Can you work these out from the model? Positions are in its coordinate system, mm. Face numbers are marked on the shaded views. A direction names the side the tool comes from. Round coordinates to 2 decimals unless told otherwise and drop trailing zeros. Write each loop counter-clockwise with the first axis right and the second up, starting at its lowest first coordinate (ties: lowest second). Pieces come first, ordered by that corner, then holes. Notation, with made-up numbers: M -38.75,-4.5 L -12.75,-4.5 A33 cw -12.75,31.5 Z; hole C -30.75,52 d6. An arc over 180 degrees is marked long. Answer in a Markdown table with one row per item. Add a question column.
(1) Suppose I cut it at C-C, the plane y = -15.25. Write out the boundary of the cut face in (x, z).
(2) For the marked faces 1, 2 and 3, which set-ups out of +Z, -Z, +X, -X, +Y, -Y let a thin tool reach every point of the face, with its end or its side?
(3) I'm going to push flat-ended pins straight in: pin 1 (8 mm diameter, centred on x = 5.5, z = -26.5, fed in from +Y); pin 2 (7 mm diameter, centred on x = -28, z = 20, fed in from +Y); pin 3 (11.5 mm diameter, centred on x = -29.5, z = -23.5, fed in from +Y); pin 4 (3 mm diameter, centred on y = -10, z = 0, fed in from +X). Where does each tip first touch, or does it pass through?
(4) Suppose I cut it at B-B, the plane x = -32. Write out the boundary of the cut face in (y, z), then the cut area to 3 significant figures.
(5) Suppose I cut it at D-D, the plane z = -13.5. Write out the boundary of the cut face in (x, y), then the cut area to 3 significant figures.
(6) Suppose I cut it at A-A, the plane x = -20. Write out the boundary of the cut face in (y, z), then the cut area to 3 significant figures.
(7) If I drill on probe 1 along Z at (x, y) = (25, -1.3); probe 2 along X at (y, z) = (-8, 1); probe 3 along X at (y, z) = (-12.75, -7), over which ranges is the centre line in solid material (lowest first)?
(8) If we mould it in two halves opening along X, with no side actions, what happens to the marked faces 4, 5 and 6? For each: released by +X, released by -X, zero draft, split by the parting line, or undercut.
from build123d import *

# Parameters (mm, degrees)
SKETCH1_W                        = 70
SKETCH1_H                        = 40
BOSS_EXTRUDE1_DEPTH              = 6.5
SKETCH2_W                        = 100
SKETCH2_H                        = 60
BOSS_EXTRUDE2_DEPTH              = 10
M3_CLEARANCE_HOLE1_D             = 3.2
SKETCH40_R                       = 3
CUT_EXTRUDE10_DEPTH              = 13.5
SKETCH7_W                        = 106.84
SKETCH7_H                        = 66.84
SKETCH7_W_2                      = 100
SKETCH7_H_2                      = 60
BOSS_EXTRUDE3_DEPTH              = 3
CUT_EXTRUDE2_DEPTH               = 1.25
M3_CLEARANCE_HOLE3_D             = 3.2
M3_CLEARANCE_HOLE3_DEPTH         = 12
M3_CLEARANCE_HOLE3_TIP           = 0.96137699
SKETCH23_W                       = 6.48
SKETCH23_H                       = 3
BOSS_EXTRUDE5_DEPTH              = 10
SKETCH26_W                       = 3.2639
SKETCH26_H                       = 13
F_1_4_CLEARANCE_HOLE2_AT_2_COUNT = 2
F_1_4_CLEARANCE_HOLE2_AT_2_PITCH = 45
SKETCH41_W                       = 35
SKETCH41_H                       = 40
SKETCH41_W_2                     = 10
SKETCH41_W_3                     = 5
CUT_EXTRUDE11_DEPTH              = 6.5
SKETCH42_W                       = 15
SKETCH42_H                       = 35
SKETCH42_W_2                     = 10
SKETCH42_H_2                     = 40
CUT_EXTRUDE12_DEPTH              = 7
CUT_EXTRUDE13_DEPTH              = 1.25
M3_CLEARANCE_HOLE5_D             = 3.2
M3_CLEARANCE_HOLE5_DEPTH         = 10
M3_CLEARANCE_HOLE5_TIP           = 0.96137699
FILLET1_R                        = 2
FILLET2_R                        = 1


with BuildPart() as part:
    # Sketch1 → Boss-Extrude1 (new body)
    with BuildSketch(Plane(origin=(0, 0, 0), x_dir=(1, 0, 0), z_dir=(0, 1, 0))):
        Rectangle(SKETCH1_W, SKETCH1_H)
    extrude(amount=-BOSS_EXTRUDE1_DEPTH)

    # Sketch2 → Boss-Extrude2 (add)
    with BuildSketch(Plane.XZ.offset(6.5)):
        with Locations((10, 0)):
            Rectangle(SKETCH2_W, SKETCH2_H)
    extrude(amount=BOSS_EXTRUDE2_DEPTH)

    # M3 Clearance Hole1 (through all)
    with Locations(Plane(origin=(0, 0, 0), x_dir=(1, 0, 0), z_dir=(0, 1, 0))):
        with Locations((-20, 7), (25, 7), (-20, -7), (25, -7)):
            Hole(M3_CLEARANCE_HOLE1_D / 2)

    # Sketch40 → Cut-Extrude10 (cut)
    with BuildSketch(Plane.XZ.offset(16.5)):
        with Locations(Location((-20, 7, 0), (0, 0, 270))):
            Circle(SKETCH40_R)
        with Locations(Location((-20, -7, 0), (0, 0, 270))):
            Circle(SKETCH40_R)
        with Locations(Location((25, 7, 0), (0, 0, 270))):
            Circle(SKETCH40_R)
        with Locations(Location((25, -7, 0), (0, 0, 270))):
            Circle(SKETCH40_R)
    extrude(amount=-CUT_EXTRUDE10_DEPTH, mode=Mode.SUBTRACT)

    # Sketch7 → Boss-Extrude3 (add)
    with BuildSketch(Plane.XZ.offset(16.5)):
        with Locations((10, 0)):
            Rectangle(SKETCH7_W, SKETCH7_H)
        with Locations((10, 0)):
            Rectangle(SKETCH7_W_2, SKETCH7_H_2, mode=Mode.SUBTRACT)
    extrude(amount=-BOSS_EXTRUDE3_DEPTH)

    # Sketch14 → Cut-Extrude2 (cut, symmetric)
    with BuildSketch(Plane.ZY.offset(36)):
        Polygon((-27.75, -8.41228676), (-27.75, -6.5), (-22.25, -6.5), (-22.25, -8.41228676), (-22.25, -11.58771324), (-25, -13.175426481), (-27.75, -11.58771324), align=None)
        Polygon((22.25, -8.41228676), (22.25, -11.58771324), (25, -13.175426481), (27.75, -11.58771324), (27.75, -8.41228676), (27.75, -6.5), (22.25, -6.5), align=None)
    extrude(amount=CUT_EXTRUDE2_DEPTH, both=True, mode=Mode.SUBTRACT)

    # M3 Clearance Hole3
    with Locations(Plane.ZY.offset(40)):
        with Locations((-25, -10), (25, -10)):
            Hole(M3_CLEARANCE_HOLE3_D / 2, depth=M3_CLEARANCE_HOLE3_DEPTH)
            with Locations((0, 0, -(M3_CLEARANCE_HOLE3_DEPTH + M3_CLEARANCE_HOLE3_TIP / 2))):  # 118° drill point
                Cone(0, M3_CLEARANCE_HOLE3_D / 2, M3_CLEARANCE_HOLE3_TIP, mode=Mode.SUBTRACT)

    # Sketch23 → Boss-Extrude5 (add, symmetric)
    with BuildSketch(Plane.XY):
        with Locations((-12, -18)):
            Rectangle(SKETCH23_W, SKETCH23_H)
    extrude(amount=BOSS_EXTRUDE5_DEPTH, both=True)

    # Sketch26 → 1/4 Clearance Hole2 (revolve, cut)
    with BuildSketch(Plane(origin=(-12, -6.5, -22.5), x_dir=(0, 0, 1), z_dir=(1, 0, 0))):
        with Locations((1.63195, 6.5)):
            Rectangle(SKETCH26_W, SKETCH26_H)
    f_1_4_clearance_hole2 = revolve(axis=Axis((-12, -0.15, -22.5), (0, -1, 0)), mode=Mode.SUBTRACT)

    # 1/4 Clearance Hole2 at 2: 1/4 Clearance Hole2 ×2
    with Locations(*[(0, 0, i * F_1_4_CLEARANCE_HOLE2_AT_2_PITCH) for i in range(1, F_1_4_CLEARANCE_HOLE2_AT_2_COUNT)]):
        add(f_1_4_clearance_hole2, mode=Mode.SUBTRACT)

    # Sketch41 → Cut-Extrude11 (cut)
    with BuildSketch(Plane(origin=(0, 0, 0), x_dir=(1, 0, 0), z_dir=(0, 1, 0))):
        with Locations((2.5, 0)):
            Rectangle(SKETCH41_W, SKETCH41_H)
        with Locations((-30, 0)):
            Rectangle(SKETCH41_W_2, SKETCH41_H)
        with Locations((32.5, 0)):
            Rectangle(SKETCH41_W_3, SKETCH41_H)
    extrude(amount=-CUT_EXTRUDE11_DEPTH, mode=Mode.SUBTRACT)

    # Sketch42 → Cut-Extrude12 (cut)
    # profile 1 of 2: a face of its own
    with BuildSketch(Plane(origin=(0, -6.5, 0), x_dir=(1, 0, 0), z_dir=(0, 1, 0))):
        with Locations((-32.5, 0)):
            Rectangle(SKETCH42_W, SKETCH42_H)
    # profile 2 of 2: a face of its own
    with BuildSketch(Plane(origin=(0, -6.5, 0), x_dir=(1, 0, 0), z_dir=(0, 1, 0))):
        Polygon((20, -30), (30, -30), (50, -30), (50, 30), (30, 30), (20, 30), (-5, 30), (-5, 17.5), (-15, 17.5), (-15, -17.5), (-5, -17.5), (-5, -30), align=None)
        with Locations((25, 0)):
            Rectangle(SKETCH42_W_2, SKETCH42_H_2, mode=Mode.SUBTRACT)
    extrude(amount=-CUT_EXTRUDE12_DEPTH, mode=Mode.SUBTRACT)

    # Sketch44 → Cut-Extrude13 (cut, symmetric)
    with BuildSketch(Plane(origin=(56, 0, 0), x_dir=(0, 0, -1), z_dir=(1, 0, 0))):
        Polygon((-2.75, -8.41228676), (-2.75, -11.58771324), (0, -13.175426481), (2.75, -11.58771324), (2.75, -8.41228676), (2.75, -6.5), (-2.75, -6.5), align=None)
    extrude(amount=CUT_EXTRUDE13_DEPTH, both=True, mode=Mode.SUBTRACT)

    # M3 Clearance Hole5
    with Locations(Plane(origin=(60, 0, 0), x_dir=(0, 0, -1), z_dir=(1, 0, 0))):
        with Locations((0, -10)):
            Hole(M3_CLEARANCE_HOLE5_D / 2, depth=M3_CLEARANCE_HOLE5_DEPTH)
            with Locations((0, 0, -(M3_CLEARANCE_HOLE5_DEPTH + M3_CLEARANCE_HOLE5_TIP / 2))):  # 118° drill point
                Cone(0, M3_CLEARANCE_HOLE5_D / 2, M3_CLEARANCE_HOLE5_TIP, mode=Mode.SUBTRACT)

    # Fillet1
    fillet1_edges = [part.edges().sort_by_distance(p)[0] for p in [
        (30, -6.75, -20),
        (30, -6.75, 20),
        (-25, -3.25, 20),
        (-25, -3.25, -20),
        (20, -6.75, 20),
        (20, -6.75, -20),
        (-15, -3.25, -20),
        (-15, -3.25, 20),
        (-25, -10, 17.5),
        (-25, -10, -17.5),
        (-40, -10, -17.5),
        (-40, -10, 17.5),
        (-15, -10, -17.5),
        (-5, -10, -17.5),
        (-5, -10, -30),
        (50, -10, -30),
        (50, -10, 30),
        (-5, -10, 30),
        (-5, -10, 17.5),
        (-15, -10, 17.5),
        (-40, -10, 30),
        (60, -10, 30),
        (60, -10, -30),
        (-40, -10, -30),
    ]]
    fillet(fillet1_edges, radius=FILLET1_R)

    # Fillet2
    fillet2_edges = [part.edges().sort_by_distance(p)[0] for p in [
        (-43.42, -15, 33.42),
        (63.42, -15, 33.42),
        (63.42, -15, -33.42),
        (-43.42, -15, -33.42),
    ]]
    fillet(fillet2_edges, radius=FILLET2_R)


solid = part.part
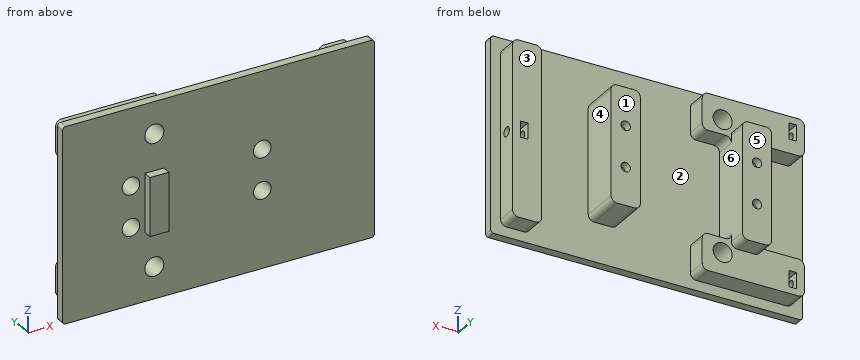
Calculated:
| question | item | result |
|---|---|---|
| 1 | outline | M -43.42,-32.42 A1 ccw -42.42,-33.42 L 62.42,-33.42 A1 ccw 63.42,-32.42 L 63.42,32.42 A1 ccw 62.42,33.42 L -42.42,33.42 A1 ccw -43.42,32.42 Z; hole C -20,-7 d6; hole C -20,7 d6; hole C -12,-22.5 d6.53; hole C -12,22.5 d6.53; hole C 25,-7 d6; hole C 25,7 d6 |
| 2 | face 1 | +Z, -Z, +X, -X, +Y |
| 2 | face 2 | +Y |
| 2 | face 3 | +Z, -Z, +X, +Y |
| 3 | pin 1 | y = -13.5 |
| 3 | pin 2 | y = 0 |
| 3 | pin 3 | y = -6.5 |
| 3 | pin 4 | x = 30 |
| 4 | outline | M -16.5,-33.42 L -13.5,-33.42 L -13.5,-30 L -6.5,-30 L -6.5,-17.5 L -13.5,-17.5 L -13.5,17.5 L -6.5,17.5 L -6.5,30 L -13.5,30 L -13.5,33.42 L -16.5,33.42 Z; hole C -10,-25 d3.2; hole C -10,25 d3.2 |
| 4 | area | 359 mm² |
| 5 | outline | M -43.42,-16.5 L 63.42,-16.5 L 63.42,-13.5 L 60,-13.5 L 60,-6.5 L 50,-6.5 L 50,-13.5 L 30,-13.5 L 30,0 L 20,0 L 20,-13.5 L -15,-13.5 L -15,0 L -25,0 L -25,-13.5 L -43.42,-13.5 Z |
| 5 | area | 661 mm² |
| 6 | outline | M -16.5,-33.42 L -13.5,-33.42 L -13.5,-30 L -6.5,-30 L -6.5,-20 L 0,-20 L 0,-8.6 L -3,-8.6 L -3,-10 L -16.5,-10 Z; M -16.5,-4 L -3,-4 L -3,-5.4 L 0,-5.4 L 0,5.4 L -3,5.4 L -3,4 L -16.5,4 Z; M -16.5,10 L -3,10 L -3,8.6 L 0,8.6 L 0,20 L -6.5,20 L -6.5,30 L -13.5,30 L -13.5,33.42 L -16.5,33.42 Z |
| 6 | area | 699 mm² |
| 7 | probe 1 | -20 to -8.6, -5.4 to 5.4, 8.6 to 20 |
| 7 | probe 2 | -25 to -15, 20 to 30, 50 to 54.75, 57.25 to 60 |
| 7 | probe 3 | -25 to -23, -17 to -15, 20 to 22, 28 to 30, 50 to 60 |
| 8 | face 4 | undercut |
| 8 | face 5 | zero draft |
| 8 | face 6 | undercut |
